The model under review builds one solid part; all positions refer to its coordinate system, in mm. Face numbers are marked on the shaded views. A direction names the side the tool comes from. Round coordinates to 2 decimals unless told otherwise and drop trailing zeros. Write each loop counter-clockwise with the first axis right and the second up, starting at its lowest first coordinate (ties: lowest second). Pieces come first, ordered by that corner, then holes. Notation, with made-up numbers: (-38, -27.75) - (-2, -27.75) arc R17 cw to (-2, -14.75) - close; hole circle Ø3 at (-16.5, 36). An arc over 180 degrees is marked (long way). One line per question, with ' | ' between items. Start each with the question number.
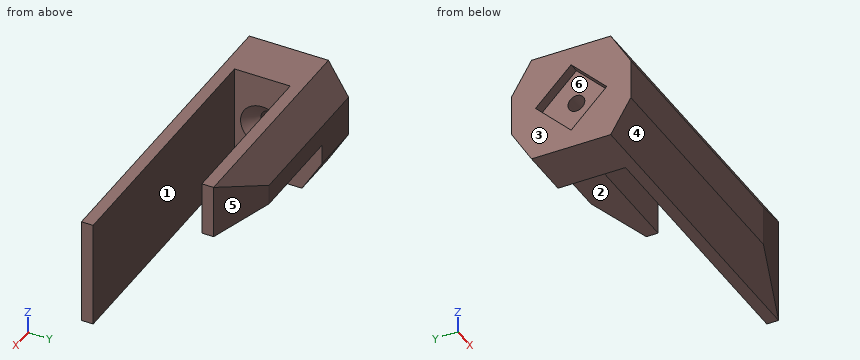
```python
from build123d import *

# Parameters (mm, degrees)
EXTRUDE_1_DEPTH     = 32
CUT_EXTRUDE_2_DEPTH = 3
SKETCH_4_R          = 2.5
CUT_EXTRUDE_3_DEPTH = 15
CHAMFER_2_SIZE      = 4
SKETCH_6_W          = 6
SKETCH_6_H          = 3.5
EXTRUDE_2_DEPTH     = 50
SKETCH_7_W          = 16
SKETCH_7_H          = 6
CUT_EXTRUDE_5_DEPTH = 50
SKETCH_8_W          = 6
SKETCH_8_H          = 3.5
EXTRUDE_3_DEPTH     = 15
SKETCH_9_W          = 15
SKETCH_9_H          = 3.5
EXTRUDE_4_DEPTH     = 6
SKETCH_10_W         = 6
SKETCH_10_H         = 3.5
EXTRUDE_5_DEPTH     = 95
SKETCH_11_W         = 65
SKETCH_11_H         = 10
SKETCH_11_W_2       = 15
CUT_EXTRUDE_6_DEPTH = 2.5
SKETCH_12_W         = 95
SKETCH_12_H         = 10
CUT_EXTRUDE_7_DEPTH = 2.5
EXTRUDE_6_DEPTH     = 95
EXTRUDE_7_DEPTH     = 65
EXTRUDE_8_DEPTH     = 15
CUT_EXTRUDE_START   = -32
CUT_EXTRUDE_9_DEPTH = 32


with BuildPart() as part:
    # Эскиз2 → Бобышка-Вытянуть1 (new body)
    with BuildSketch(Plane.XY):
        Polygon((0, 0), (65, 0), (65, -6), (15, -6), (15, -22.6), (95, -22.6), (95, -28.6), (0, -28.6), align=None)
    extrude(amount=EXTRUDE_1_DEPTH)

    # Эскиз3 → Вырез-Вытянуть2 (cut)
    with BuildSketch(Plane.ZY):
        Polygon((5.393398282, -14.3), (16, -24.906601718), (26.606601718, -14.3), (16, -3.693398282), align=None)
    extrude(amount=-CUT_EXTRUDE_2_DEPTH, mode=Mode.SUBTRACT)

    # Эскиз4 → Вырез-Вытянуть3 (cut)
    with BuildSketch(Plane.ZY):
        with Locations(Location((16, -14.3, 0), (0, 0, 270))):
            Circle(SKETCH_4_R)
    extrude(amount=-CUT_EXTRUDE_3_DEPTH, mode=Mode.SUBTRACT)

    # Фаска2
    chamfer_2_edges = [part.edges().sort_by_distance(p)[0] for p in [
        (15, -11.8, 16),
    ]]
    chamfer(chamfer_2_edges, length=CHAMFER_2_SIZE)

    # Эскиз6 → Бобышка-Вытянуть2 (add)
    with BuildSketch(Plane(origin=(65, 0, 0), x_dir=(0, 0, -1), z_dir=(1, 0, 0))):
        with Locations((-19, 1.75)):
            Rectangle(SKETCH_6_W, SKETCH_6_H)
    extrude(amount=-EXTRUDE_2_DEPTH)

    # Эскиз7 → Вырез-Вытянуть5 (cut)
    with BuildSketch(Plane(origin=(65, 0, 0), x_dir=(0, 0, -1), z_dir=(1, 0, 0))):
        with Locations((-8, -3)):
            Rectangle(SKETCH_7_W, SKETCH_7_H)
    extrude(amount=-CUT_EXTRUDE_5_DEPTH, mode=Mode.SUBTRACT)

    # Эскиз8 → Бобышка-Вытянуть3 (add)
    with BuildSketch(Plane.ZY.offset(-15)):
        with Locations((19, 1.75)):
            Rectangle(SKETCH_8_W, SKETCH_8_H)
    extrude(amount=EXTRUDE_3_DEPTH)

    # Эскиз9 → Бобышка-Вытянуть4 (add)
    with BuildSketch(Plane(origin=(0, 0, 16), x_dir=(-1, 0, 0), z_dir=(0, 0, -1))):
        with Locations((-7.5, 1.75)):
            Rectangle(SKETCH_9_W, SKETCH_9_H)
    extrude(amount=EXTRUDE_4_DEPTH)

    # Эскиз10 → Бобышка-Вытянуть5 (add)
    with BuildSketch(Plane.ZY):
        with Locations((13, -30.35)):
            Rectangle(SKETCH_10_W, SKETCH_10_H)
        with Locations((19, -30.35)):
            Rectangle(SKETCH_10_W, SKETCH_10_H)
    extrude(amount=-EXTRUDE_5_DEPTH)

    # Эскиз11 → Вырез-Вытянуть6 (cut)
    with BuildSketch(Plane(origin=(0, 0, 0), x_dir=(1, 0, 0), z_dir=(0, 1, 0))):
        with Locations((32.5, -27)):
            Rectangle(SKETCH_11_W, SKETCH_11_H)
        with Locations((7.5, -5)):
            Rectangle(SKETCH_11_W_2, SKETCH_11_H)
    extrude(amount=-CUT_EXTRUDE_6_DEPTH, mode=Mode.SUBTRACT)

    # Эскиз12 → Вырез-Вытянуть7 (cut)
    with BuildSketch(Plane.XZ.offset(28.6)):
        with Locations((47.5, 5)):
            Rectangle(SKETCH_12_W, SKETCH_12_H)
        with Locations((47.5, 27)):
            Rectangle(SKETCH_12_W, SKETCH_12_H)
    extrude(amount=-CUT_EXTRUDE_7_DEPTH, mode=Mode.SUBTRACT)

    # Эскиз13 → Бобышка-Вытянуть6 (add)
    with BuildSketch(Plane.ZY):
        Polygon((0, -26.1), (10, -32.1), (10, -26.1), align=None)
        Polygon((22, -26.1), (22, -32.1), (32, -26.1), align=None)
    extrude(amount=-EXTRUDE_6_DEPTH)

    # Эскиз14 → Бобышка-Вытянуть7 (add)
    with BuildSketch(Plane.ZY):
        Polygon((22, 3.5), (32, -2.5), (22, -2.5), align=None)
    extrude(amount=-EXTRUDE_7_DEPTH)

    # Эскиз15 → Бобышка-Вытянуть8 (add)
    with BuildSketch(Plane.ZY):
        Polygon((10, 3.5), (10, -2.5), (0, -2.5), align=None)
    extrude(amount=-EXTRUDE_8_DEPTH)

    # Эскиз16 → Вырез-Вытянуть9 (cut)
    with BuildSketch(Plane.XY.offset(32).offset(CUT_EXTRUDE_START)):
        Polygon((65, -2.5), (65, 3.5), (45, 3.5), align=None)
        Polygon((95, -26.1), (95, -32.1), (75, -32.1), align=None)
    extrude(amount=CUT_EXTRUDE_9_DEPTH, mode=Mode.SUBTRACT)


solid = part.part
```
1. Add section D-D, the plane y = -5. Write out the cut boundary in (x, z).
2. Add section B-B, the plane z = 6.5. Write out the cut boundary in (x, y).
3. The part is to be moulded in two halves that separate along Y. For the marked faces 4, 5 and 6, say which applies: pulls with the +Y half, pulls with the -Y half, needs draft (parallel to the pull), parting line crosses it, or undercut.
4. Machinability: for the marked faces 1, 2 and 3, which of the approach directions +Z, -Z, +X, -X, +Y, -Y give a long, thin tool a straight path to every point of the face, cutting with its end or side? Answer none if there is none.
5. Add section A-A, the plane x = 38. Write out the cut boundary in (y, z).
6. Add section C-C, the plane y = -27. Write out the cut boundary in (x, z), then the cut area to 3 significant figures.
7. Clearance check with flat-ended pins moving along their axes: P1, Ø3, axis at x = 45.5, y = -1.5, coming from the -Z side; P2, Ø1.5, axis at x = 75, y = -24.5, coming from the -Z side; P3, Ø3, axis at x = 14, z = 25.5, coming from the +Y side; P4, Ø8, axis at x = 31, z = 26.5, coming from the -Y side. State where each tip first meets the part, or that it passes through.
8. Wall thickness on line 1 along Z through (x, y) = (7.5, -14.3); line 2 along Y through (x, z) = (33, 21.5); line 3 along Z through (x, y) = (39, -5.5): over which ranges is each line inside the solid? List them lowest first. Write a range as [from, to].
Geometry check:
1) outline: (0, 0) - (15, 0) - (15, 16) - (65, 16) - (65, 32) - (0, 32) - (0, 17.31) - (3, 17.31) - (3, 14.69) - (0, 14.69) - close
2) outline: (0, -30) - (82, -30) - (95, -26.1) - (95, -22.6) - (15, -22.6) - (15, 1.4) - (0, 1.4) - (0, -13.19) - (3, -13.19) - (3, -15.41) - (0, -15.41) - close
3) face 4: pulls with the -Y half | face 5: pulls with the +Y half | face 6: undercut
4) face 1: +Z, -Z, +X | face 2: -Z, +X, +Y | face 3: +Z, -Z, -X, +Y, -Y
5) outline: (-32.1, 10) - (-26.1, 0) - (-22.6, 0) - (-22.6, 32) - (-26.1, 32) - (-32.1, 22) - close; (-6, 16) - (3.5, 16) - (3.5, 22) - (-2.5, 32) - (-6, 32) - close
6) outline: (0, 1.5) - (92, 1.5) - (92, 30.5) - (0, 30.5) - close | area: 2,670 mm2
7) P1: stops at z = 16 | P2: stops at z = 0 | P3: stops at y = 2.3 | P4: stops at y = -31.8
8) line 1: z = [0, 13.5], [18.5, 32] | line 2: y = [-32.1, -22.6], [-6, 3.5] | line 3: z = [16, 32]
